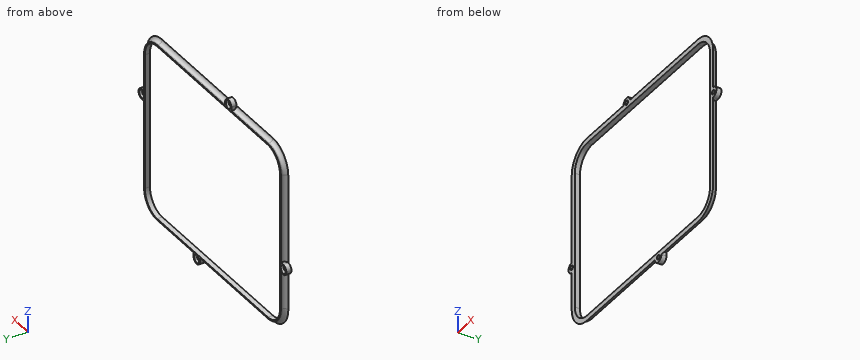
from build123d import *

# Parameters (mm, degrees)
BOSS_EXTRUDE1_DEPTH                             = 4
SKETCH2_R                                       = 1.6
BOSS_EXTRUDE2_DEPTH                             = 4
CSK_FOR_M3_FLAT_HEAD_MACHINE_SCREW1_D           = 3.4
CSK_FOR_M3_FLAT_HEAD_MACHINE_SCREW1_CSINK_D     = 6.3
CSK_FOR_M3_FLAT_HEAD_MACHINE_SCREW1_CSINK_ANGLE = 90


with BuildPart() as part:
    # Sketch1 → Boss-Extrude1 (new body)
    with BuildSketch(Plane(origin=(0, 0, 0), x_dir=(1, 0, 0), z_dir=(0, 1, 0))):
        with BuildLine():
            Line((86.7, -53.6), (86.7, 53.6))
            ThreePointArc((86.7, 53.6), (81.86726189, 65.26726189), (70.2, 70.1))
            Line((70.2, 70.1), (-70.2, 70.1))
            ThreePointArc((-70.2, 70.1), (-81.86726189, 65.26726189), (-86.7, 53.6))
            Line((-86.7, 53.6), (-86.7, -53.6))
            ThreePointArc((-86.7, -53.6), (-81.86726189, -65.26726189), (-70.2, -70.1))
            Line((-70.2, -70.1), (70.2, -70.1))
            ThreePointArc((70.2, -70.1), (81.86726189, -65.26726189), (86.7, -53.6))
        make_face()
        with BuildLine():
            Line((-70.2, -69.1), (70.2, -69.1))
            ThreePointArc((70.2, -69.1), (81.160155108, -64.560155108), (85.7, -53.6))
            Line((85.7, -53.6), (85.7, 53.6))
            ThreePointArc((85.7, 53.6), (81.160155108, 64.560155108), (70.2, 69.1))
            Line((70.2, 69.1), (-70.2, 69.1))
            ThreePointArc((-70.2, 69.1), (-81.160155108, 64.560155108), (-85.7, 53.6))
            Line((-85.7, 53.6), (-85.7, -53.6))
            ThreePointArc((-85.7, -53.6), (-81.160155108, -64.560155108), (-70.2, -69.1))
        make_face(mode=Mode.SUBTRACT)
    extrude(amount=BOSS_EXTRUDE1_DEPTH)

    # Sweep1: sweep along a path in Sketch5
    with BuildLine(Plane.XZ) as sweep1_path:
        Line((86.7, 53.6), (86.7, -53.6))
        ThreePointArc((86.7, -53.6), (81.86726189, -65.26726189), (70.2, -70.1))
        Line((70.2, -70.1), (-70.2, -70.1))
        ThreePointArc((-70.2, -70.1), (-81.86726189, -65.26726189), (-86.7, -53.6))
        Line((-86.7, -53.6), (-86.7, 53.6))
        ThreePointArc((-86.7, 53.6), (-81.86726189, 65.26726189), (-70.2, 70.1))
        Line((-70.2, 70.1), (70.2, 70.1))
        ThreePointArc((70.2, 70.1), (81.86726189, 65.26726189), (86.7, 53.6))
    # Sketch4 → Sweep1 (sweep)
    with BuildSketch(Plane.XY):
        with BuildLine():
            Line((-86.7, 0), (-89.7, 0))
            ThreePointArc((-89.7, 0), (-87.578679656, 0.878679656), (-86.7, 3))
            Line((-86.7, 3), (-86.7, 0))
        make_face()
    sweep(path=sweep1_path.line)

    # Sketch2 → Boss-Extrude2 (add, through all)
    # profile 1 of 4: a face of its own
    with BuildSketch(Plane(origin=(0, 0, 0), x_dir=(1, 0, 0), z_dir=(0, 1, 0))):
        with BuildLine():
            Line((-86.7, 24), (-89.7, 24))
            ThreePointArc((-89.7, 24), (-93.7, 20), (-89.7, 16))
            Line((-89.7, 16), (-86.7, 16))
            Line((-86.7, 16), (-86.7, 24))
        make_face()
        with Locations(Location((-89.7, 20, 0), (0, 0, 270))):
            Circle(SKETCH2_R, mode=Mode.SUBTRACT)
    # profile 2 of 4: a face of its own
    with BuildSketch(Plane(origin=(0, 0, 0), x_dir=(1, 0, 0), z_dir=(0, 1, 0))):
        with BuildLine():
            Line((16, 70.1), (16, 73.1))
            ThreePointArc((16, 73.1), (20, 77.1), (24, 73.1))
            Line((24, 73.1), (24, 70.1))
            Line((24, 70.1), (16, 70.1))
        make_face()
        with Locations((20, 73.1)):
            Circle(SKETCH2_R, mode=Mode.SUBTRACT)
    # profile 3 of 4: a face of its own
    with BuildSketch(Plane(origin=(0, 0, 0), x_dir=(1, 0, 0), z_dir=(0, 1, 0))):
        with BuildLine():
            Line((-24, -70.1), (-24, -73.1))
            ThreePointArc((-24, -73.1), (-20, -77.1), (-16, -73.1))
            Line((-16, -73.1), (-16, -70.1))
            Line((-16, -70.1), (-24, -70.1))
        make_face()
        with Locations(Location((-20, -73.1, 0), (0, 0, 180))):
            Circle(SKETCH2_R, mode=Mode.SUBTRACT)
    # profile 4 of 4: a face of its own
    with BuildSketch(Plane(origin=(0, 0, 0), x_dir=(1, 0, 0), z_dir=(0, 1, 0))):
        with BuildLine():
            Line((86.7, -24), (89.7, -24))
            ThreePointArc((89.7, -24), (93.7, -20), (89.7, -16))
            Line((89.7, -16), (86.7, -16))
            Line((86.7, -16), (86.7, -24))
        make_face()
        with Locations(Location((89.7, -20, 0), (0, 0, 270))):
            Circle(SKETCH2_R, mode=Mode.SUBTRACT)
    extrude(amount=BOSS_EXTRUDE2_DEPTH)

    # CSK for M3 Flat Head Machine Screw1 (through all)
    with Locations(Plane(origin=(20, 4, -73.1), x_dir=(0, 0, 1), z_dir=(0, 1, 0))):
        with Locations((0, 0), (53.1, -109.7), (93.1, 69.7), (146.2, -40)):
            CounterSinkHole(CSK_FOR_M3_FLAT_HEAD_MACHINE_SCREW1_D / 2, CSK_FOR_M3_FLAT_HEAD_MACHINE_SCREW1_CSINK_D / 2, counter_sink_angle=CSK_FOR_M3_FLAT_HEAD_MACHINE_SCREW1_CSINK_ANGLE)


solid = part.part
Read the model definition and answer for the solid it produces. Units are mm, in the model's axes. Give positions to 0.01 mm unless a question says otherwise; leave off trailing zeros. Write each loop counter-clockwise with the first axis right and the second up, starting at its lowest first coordinate (ties: lowest second). Pieces come first, ordered by that corner, then holes. Notation, with made-up numbers: (-6.75, -6) - (2.25, -6) arc R33 cw to (2.25, 27) - close; hole circle Ø6 at (72, -4.75). An arc over 180 degrees is marked (long way). Answer in a Markdown table with one row per item. Add a question column.
Item 1: Section A-A, the plane z = 38 is taken. Write down the section's boundary in (x, y).
Item 2: Section B-B, the plane x = -11.5 is taken. Write down the section's boundary in (y, z).
Item 3: Find the intervals of material crossed by L1, parallel to Z at x = 20, y = 0.5; L2, parallel to X at y = 2.7, z = -33; L3, parallel to Z at x = 36.5, y = 3.6, in increasing order.
Item 4: Flat-ended cylindrical pins translate along their axes: P1, Ø0.9, axis at y = 1, z = 72, coming from the -X side; P2, Ø1.1, axis at y = 3.5, z = -9.5, coming from the +X side; P3, Ø0.5, axis at x = -33.5, y = 3.5, coming from the -Z side. Find the tip coordinate at first contact, or state that the pin passes through.
Recorded:
| question | item | result |
|---|---|---|
| 1 | outline | (-89.7, 0) - (-85.7, 0) - (-85.7, 4) - (-86.7, 4) - (-86.7, 3) arc R3 cw to start; (85.7, 0) - (89.7, 0) arc R3 cw to (86.7, 3) - (86.7, 4) - (85.7, 4) - close |
| 2 | outline | (0, -73.1) arc R3 cw to (3, -70.1) - (4, -70.1) - (4, -69.1) - (0, -69.1) - close; (0, 69.1) - (4, 69.1) - (4, 70.1) - (3, 70.1) arc R3 cw to (0, 73.1) - close |
| 3 | L1 | z = -77.1 to -74.8, -71.4 to -69.1, 69.1 to 71.44 |
| 3 | L2 | x = -86.72 to -85.7, 85.7 to 86.72 |
| 3 | L3 | z = -70.1 to -69.1, 69.1 to 70.1 |
| 4 | P1 | stops at x = -24 |
| 4 | P2 | stops at x = 86.7 |
| 4 | P3 | stops at z = -70.1 |
